Here's how the part is built. I have some questions about the finished solid (model axes, mm). Coordinates: 2 decimals unless noted, no trailing zeros. Order: outer loops, then holes, each group sorted by start corner. A loop starts at its lowest first (then second) coordinate and runs counter-clockwise, first axis right, second up. Notation, with made-up numbers: (-38, -14.75) - (-31, -14.75) arc R31 ccw to (-31, 16.25) - close; hole circle Ø10 at (79, -35.5). An arc over 180 degrees is marked (long way). Answer in a Markdown table with one row per item. Add a question column.
Item 1: I want a section at A-A (z = 35). Please give me the cut outline in (x, y), plus the area to 3 significant figures.
Item 2: Will these pins go through, and if not, where does the flat tip stop? pin 1 Ø3 at (x, z) = (-35, -35) entering from -Y; pin 2 Ø5 at (x, z) = (9.55, 9.55) entering from -Y.
Item 3: I want a section at D-D (x = -4). Please give me the cut outline in (y, z).
Item 4: I want a section at B-B (y = -0.5). Count the separate pieces of the cut face and the enclosed holes in it, plus the area to 3 significant figures.
Item 5: If I drill on line 1 along X through (y, z) = (-0.1, 35); line 2 along X through (y, z) = (0.1, -9.55), over which ranges is the centre line in solid material (lowest first)? Write a range as from..to.
Item 6: I want a section at C-C (x = 9.55). Please give me the cut outline in (y, z).
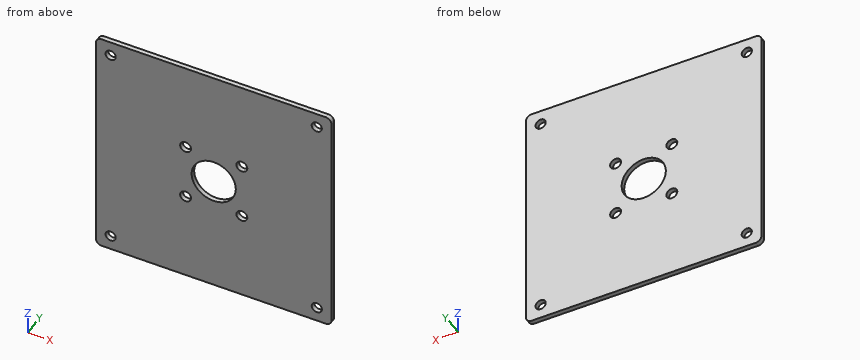
Autodesk Inventor part; units mm, degrees
ref_plane "YZ Plane" through (0, 0, 0) normal (1, 0, 0) x (0, 1, 0)
ref_plane "XZ Plane" through (0, 0, 0) normal (0, 1, 0) x (-1, 0, 0)
ref_plane "XY Plane" through (0, 0, 0) normal (0, 0, 1) x (1, 0, 0)
sketch "Sketch1" plane through (0, 0, 0) normal (0, 1, 0) x (-1, 0, 0)
  line L0 (40, -40) -> (-40, -40)
  line L1 (-40, -40) -> (-40, 40)
  line L2 (-40, 40) -> (40, 40)
  line L3 (40, 40) -> (40, -40)
  point P0 (0, 0)
  point P1 (0, -40)
  point P2 (-40, 0)
  dimension "d15" = 80
  dimension "d16" = 80
extrude "Extrusion1" add sketch "Sketch1" along normal mid plane 1.6
fillet "Fillet1" radius 2 4 edges at (-40, 0, 40) (40, 0, 40) (40, 0, -40) (-40, 0, -40)
sketch "Sketch2" plane through (0, 0.8, 0) normal (0, 1, 0) x (1, 0, 0)
  line L0 (0, 0) -> (-7.9877, 0) construction
  line L1 (0, 0) -> (0, 5.5351) construction
  point P0 (-35, -35)
  point P1 (-35, 35)
  point P2 (35, -35)
  point P3 (35, 35)
  dimension "d18" = 35
  dimension "d19" = 35
hole "Hole1" at (-35, 0.8, 35) at (-35, 0.8, -35) at (35, 0.8, 35) at (35, 0.8, -35) direction (0, -1, 0) diameter 3.454 end through all
sketch "Sketch3" plane through (0, 0.8, 0) normal (0, 1, 0) x (1, 0, 0)
  line L0 (-12.55, 12.55) -> (12.55, 12.55)
  line L1 (12.55, 12.55) -> (12.55, -12.55)
  line L2 (12.55, -12.55) -> (-12.55, -12.55)
  line L3 (-12.55, -12.55) -> (-12.55, 12.55)
  line L4 (0, 0) -> (0, 3.6765) construction
  line L5 (0, 0) -> (3.2883, 0) construction
  point P0 (12.55, 0)
  point P1 (0, 12.55)
  point P2 (-9.55, 9.55)
  point P3 (9.55, 9.55)
  point P4 (-9.55, -9.55)
  point P5 (9.55, -9.55)
  dimension "d27" = 25.1
  dimension "d28" = 25.1
  dimension "d29" = 3
  dimension "d30" = 3
hole "Hole2" at (-9.55, 0.8, -9.55) at (9.55, 0.8, -9.55) at (-9.55, 0.8, 9.55) at (9.55, 0.8, 9.55) direction (0, -1, 0) diameter 3.7 end through all
sketch "Sketch4" plane through (0, 0.8, 0) normal (0, 1, 0) x (1, 0, 0)
  circle A0 centre (0, 0) radius 7.5
  dimension "d38" = 15
extrude "Extrusion2" cut sketch "Sketch4" against normal through all
properties part number "pcb"
Values follow:
| question | item | result |
|---|---|---|
| 1 | outline | (-40, -0.8) - (-36.73, -0.8) - (-36.73, 0.8) - (-40, 0.8) - close; (-33.27, -0.8) - (33.27, -0.8) - (33.27, 0.8) - (-33.27, 0.8) - close; (36.73, -0.8) - (40, -0.8) - (40, 0.8) - (36.73, 0.8) - close |
| 1 | area | 117 mm^2 |
| 2 | pin 1 | passes through |
| 2 | pin 2 | stops at y = -0.8 |
| 3 | outline | (-0.8, -40) - (0.8, -40) - (0.8, -6.34) - (-0.8, -6.34) - close; (-0.8, 6.34) - (0.8, 6.34) - (0.8, 40) - (-0.8, 40) - close |
| 4 | separate pieces | 1 |
| 4 | enclosed holes | 9 |
| 4 | area | 6,140 mm^2 |
| 5 | line 1 | x = -40..-36.73, -33.27..33.27, 36.73..40 |
| 5 | line 2 | x = -40..-11.4, -7.7..7.7, 11.4..40 |
| 6 | outline | (-0.8, -40) - (0.8, -40) - (0.8, -11.4) - (-0.8, -11.4) - close; (-0.8, -7.7) - (0.8, -7.7) - (0.8, 7.7) - (-0.8, 7.7) - close; (-0.8, 11.4) - (0.8, 11.4) - (0.8, 40) - (-0.8, 40) - close |
